Could you check a few things on this model? Use its own coordinates, in mm. Give positions to 0.01 mm unless a question says otherwise; leave off trailing zeros. Write each loop counter-clockwise with the first axis right and the second up, starting at its lowest first coordinate (ties: lowest second). Pieces come first, ordered by that corner, then holes. Notation, with made-up numbers: (46.5, 55.5) -> (54.5, 55.5) arc R17 cw to (54.5, 84.5) -> close; hole circle Ø9 at (-22.5, 27.25). An arc over 180 degrees is marked (long way). One line per question, with ' | ' between items.
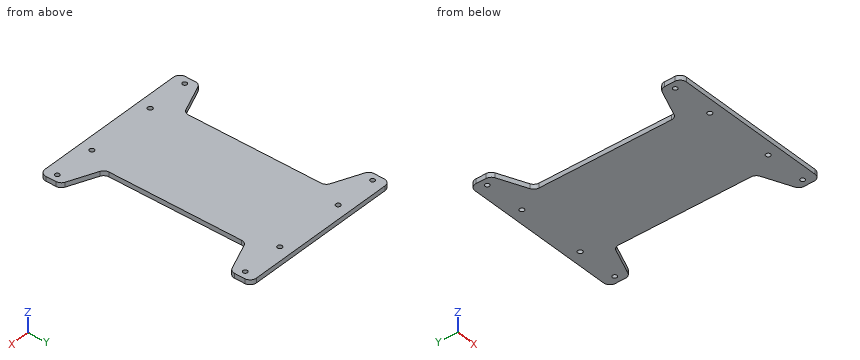
Autodesk Inventor part; units mm, degrees
ref_plane "YZ Plane" through (0, 0, 0) normal (1, 0, 0) x (0, 1, 0)
ref_plane "XZ Plane" through (0, 0, 0) normal (0, 1, 0) x (-1, 0, 0)
ref_plane "XY Plane" through (0, 0, 0) normal (0, 0, 1) x (1, 0, 0)
sketch "Sketch1" plane through (0, 0, 0) normal (0, 0, 1) x (1, 0, 0)
  point P0 (0, 0)
sketch "Sketch2" plane through (0, 0, 0) normal (0, 0, 1) x (1, 0, 0)
  line L0 (-52.4998, -67.5002) -> (52.4998, -67.5002)
  line L1 (52.4998, -67.5002) -> (52.4998, 67.5002)
  line L2 (52.4998, 67.5002) -> (-52.4998, 67.5002)
  line L3 (-52.4998, 67.5002) -> (-52.4998, -67.5002)
  circle A0 centre (22, 60) radius 1.4999
  circle A1 centre (-22, 60) radius 1.4999
  circle A2 centre (22, -60) radius 1.4999
  circle A3 centre (-22, -60) radius 1.4999
  line L4 (0, -44.9999) -> (0, 44.9999)
  line L5 (30, -44.9999) -> (30, 44.9999)
  line L6 (30, 44.9999) -> (52.4998, 54.3179)
  line L7 (30, -44.9999) -> (52.4998, -54.3208)
  line L8 (-30, -44.9999) -> (-30, 44.9999)
  line L9 (-30, 44.9999) -> (-52.4998, 54.3179)
  line L10 (-30, -44.9999) -> (-52.4998, -54.3208)
  circle A4 centre (0, 0) radius 1.4203
  circle A5 centre (48, 60) radius 1.4203
  circle A6 centre (-48, 60) radius 1.4203
  circle A7 centre (48, -60) radius 1.4203
  circle A8 centre (-48, -60) radius 1.4203
extrude "Extrusion3" add sketch "Sketch2" along normal blind 3 contours L3 L10 L8 L9 L2 L1 L6 L5 L7 L0 | L3 L9 L8 L10 | L7 L5 L6 L1 | A4 L4 | L4 A4 | A5 | A6 | A7 | A8
fillet "Fillet4" radius 4 4 edges at (-52.4998, 67.5002, 1.5) (52.4998, 67.5002, 1.5) (52.4998, -67.5002, 1.5) (-52.4998, -67.5002, 1.5)
extrude "Extrusion4" cut sketch "Sketch2" along normal blind 10 contours L3 L9 L8 L10 | L7 L5 L6 L1
fillet "Fillet5" radius 4 8 edges at (52.4998, 54.3179, 1.5) (30, 44.9999, 1.5) (-30, 44.9999, 1.5) (-52.4998, 54.3179, 1.5) (-30, -44.9999, 1.5) (-52.4998, -54.3208, 1.5) (30, -44.9999, 1.5) (52.4998, -54.3208, 1.5)
extrude "Extrusion5" cut sketch "Sketch2" along normal blind 10 contours A5 | A6 | A7 | A8
properties part number "Controller - Power Board v2"
Q1. Will these pins go through, and if not, where does the flat tip stop? pin 1 (1.5 mm diameter, centred on y = 6.5, z = 1.5, fed in from +X); pin 2 (1 mm diameter, centred on y = 44.5, z = 2.5, fed in from -X); pin 3 (0.9 mm diameter, centred on y = 8, z = 2, fed in from -X).
Answer below:
pin 1: stops at x = 30 | pin 2: stops at x = -31.02 | pin 3: stops at x = -30
Q2. Imagine slicing it at D-D on y = -35. Please give me the cut outline in (x, z), and give its area (3 significant figures).
Answer below:
outline: (-30, 0) -> (30, 0) -> (30, 3) -> (-30, 3) -> close | area: 180 mm^2
Q3. Imagine slicing it at B-B on x = 22. Please give me the cut outline in (y, z), and give its area (3 significant figures).
Answer below:
outline: (-67.5, 0) -> (-61.5, 0) -> (-61.5, 3) -> (-67.5, 3) -> close; (-58.5, 0) -> (58.5, 0) -> (58.5, 3) -> (-58.5, 3) -> close; (61.5, 0) -> (67.5, 0) -> (67.5, 3) -> (61.5, 3) -> close | area: 387 mm^2
Q4. If I drill on line 1 along Y through (x, z) = (-22.5, 0.4); line 2 along Y through (x, z) = (22, 2.35); line 3 along X through (y, z) = (24.5, 2.15), over which ranges is the centre line in solid material (lowest first)?
Answer below:
line 1: y = -67.5 to -61.41, -58.59 to 58.59, 61.41 to 67.5 | line 2: y = -67.5 to -61.5, -58.5 to 58.5, 61.5 to 67.5 | line 3: x = -30 to 30
Q5. Imagine slicing it at C-C on z = 2.25. Count the separate pieces of the cut face and the enclosed holes in it, and give its area (3 significant figures).
Answer below:
separate pieces: 1 | enclosed holes: 8 | area: 9,640 mm^2
Q6. Imagine slicing it at A-A on y = 60. Please give me the cut outline in (x, z).
Answer below:
outline: (-52.5, 0) -> (-49.42, 0) -> (-49.42, 3) -> (-52.5, 3) -> close; (-46.58, 0) -> (-23.5, 0) -> (-23.5, 3) -> (-46.58, 3) -> close; (-20.5, 0) -> (20.5, 0) -> (20.5, 3) -> (-20.5, 3) -> close; (23.5, 0) -> (46.58, 0) -> (46.58, 3) -> (23.5, 3) -> close; (49.42, 0) -> (52.5, 0) -> (52.5, 3) -> (49.42, 3) -> close
